from build123d import *

# Parameters (mm, degrees)
F1_DEPTH = 57.15
F2_R     = 10.3251
F3_DEPTH = 7.9375
F4_R     = 9.92251
F5_DEPTH = 88.9


with BuildPart() as f1:
    # F0 (on Right) → F1 (new body)
    with BuildSketch(Plane.YZ):
        with BuildLine():
            Line((-31.75, 0), (0, 0))
            Line((0, 0), (31.75, 0))
            ThreePointArc((31.75, 0), (40.730256, 3.719744), (44.45, 12.7))
            Line((44.45, 12.7), (44.45, 73.025))
            Line((44.45, 73.025), (36.5125, 73.025))
            Line((36.5125, 73.025), (36.5125, 12.7))
            ThreePointArc((36.5125, 12.7), (35.117596, 9.332404), (31.75, 7.9375))
            Line((31.75, 7.9375), (-31.75, 7.9375))
            ThreePointArc((-31.75, 7.9375), (-35.117596, 9.332404), (-36.5125, 12.7))
            Line((-36.5125, 12.7), (-36.5125, 73.025))
            Line((-36.5125, 73.025), (-44.45, 73.025))
            Line((-44.45, 73.025), (-44.45, 12.7))
            ThreePointArc((-44.45, 12.7), (-40.730256, 3.719744), (-31.75, 0))
        make_face()
    extrude(amount=F1_DEPTH)

    # F2 (on face) → F3 (join)
    with BuildSketch(Plane.XY.offset(7.9375)):
        with BuildLine():
            ThreePointArc((63.5, 22.225), (59.009872, 24.084872), (57.15, 28.575))
            Line((57.15, 28.575), (57.15, -28.575))
            ThreePointArc((57.15, -28.575), (59.009872, -24.084872), (63.5, -22.225))
            Line((63.5, -22.225), (111.125, -22.225))
            ThreePointArc((111.125, -22.225), (133.35, 0), (111.125, 22.225))
            Line((111.125, 22.225), (63.5, 22.225))
        make_face()
        with Locations((73.025, 0)):
            Circle(F2_R, mode=Mode.SUBTRACT)
        with Locations((111.125, 0)):
            Circle(F2_R, mode=Mode.SUBTRACT)
    extrude(amount=-F3_DEPTH)

    # F4 (on face) → F5 (cut)
    with BuildSketch(Plane.XZ.offset(44.45)):
        with Locations((28.575, 44.45)):
            Circle(F4_R)
        with BuildLine():
            Line((28.575, 73.025), (0, 73.025))
            Line((0, 73.025), (0, 44.45))
            ThreePointArc((0, 44.45), (8.369424, 64.655576), (28.575, 73.025))
        make_face()
        with BuildLine():
            Line((57.15, 73.025), (28.575, 73.025))
            ThreePointArc((28.575, 73.025), (48.780576, 64.655576), (57.15, 44.45))
            Line((57.15, 44.45), (57.15, 73.025))
        make_face()
    extrude(amount=-F5_DEPTH, mode=Mode.SUBTRACT)


solid = f1.part
Could you check a few things on this model? Use its own coordinates, in mm. A direction names the side the tool comes from. Round coordinates to 2 decimals unless told otherwise and drop trailing zeros. Write each loop counter-clockwise with the first axis right and the second up, starting at its lowest first coordinate (ties: lowest second). Pieces come first, ordered by that corner, then holes. Notation, with made-up numbers: (-26.75, 75.25) -> (32.25, 75.25) arc R13 ccw to (32.25, 82.25) -> close; hole circle Ø7 at (7.25, 61.5). An arc over 180 degrees is marked (long way). Use a Markdown table: item, result.
1. We'd pull the mould along Y, two halves only. Please class faces 4 (the face through (21.8, -44.45, 36.6)), 5 (the face through (22, 44.45, 36)), 6 (the face through (0, -0.6, 7.7)), 7 (the face through (22, -36.512, 36)): +Y half, -Y half, draft (parallel to the pull), parting line (faces both ways), or undercut.
Answer key:
| item | result |
|---|---|
| face 4 | -Y half |
| face 5 | +Y half |
| face 6 | draft |
| face 7 | undercut |
2. If we section it at A-A (z = 22.5): List the corners of the cut face in (x, y) for me, then the cut area to 3 significant figures.
Answer key:
| item | result |
|---|---|
| outline | (0, -44.45) -> (57.15, -44.45) -> (57.15, -36.51) -> (0, -36.51) -> close; (0, 36.51) -> (57.15, 36.51) -> (57.15, 44.45) -> (0, 44.45) -> close |
| area | 907 mm^2 |
3. If we section it at C-C (x = 67.5): List the corners of the cut face in (y, z) for me (1 decimal).
Answer key:
| item | result |
|---|---|
| outline | (-22.2, 0) -> (-8.7, 0) -> (-8.7, 7.9) -> (-22.2, 7.9) -> close; (8.7, 0) -> (22.2, 0) -> (22.2, 7.9) -> (8.7, 7.9) -> close |
4. If we section it at D-D (x = 32): State how many separate pieces and enclosed holes the cut face has, then the cut area to 3 significant figures.
Answer key:
| item | result |
|---|---|
| separate pieces | 3 |
| enclosed holes | 0 |
| area | 1,380 mm^2 |
5. If we section it at B-B (y = 0): List the corners of the cut face in (x, z) for me.
Answer key:
| item | result |
|---|---|
| outline | (0, 0) -> (62.7, 0) -> (62.7, 7.94) -> (0, 7.94) -> close; (83.35, 0) -> (100.8, 0) -> (100.8, 7.94) -> (83.35, 7.94) -> close; (121.45, 0) -> (133.35, 0) -> (133.35, 7.94) -> (121.45, 7.94) -> close |
6. Which directions (+Z, -Z, +X, -X, +Y, -Y) give clear straight access to the entire face, cutting with the end or side of a thin tool? Please do faces 1 (the face through (57.15, 38, 23)), 2 (the face through (57.15, -38, 23)), 3 (the face through (28.175, 35.154, 9.37)).
Answer key:
| item | result |
|---|---|
| face 1 | +Z, -Z, +X, +Y |
| face 2 | +Z, -Z, +X, -Y |
| face 3 | +Z, +X, -X |
7. For pin 1 Ø17.5 at (y, z) = (-36, 12.5) entering from +X; pin 2 Ø4 at (x, z) = (78.5, 4.5) entering from -Y (3 decimals); pin 3 Ø12 at (x, y) = (102, -16) entering from -Z; pin 4 Ø4 at (x, y) = (80.5, 7.5) entering from +Z, each with a flat end and sliding along its axis, tell me the tip position at first contact or that it passes through.
Answer key:
| item | result |
|---|---|
| pin 1 | stops at x = 57.15 |
| pin 2 | stops at y = -22.225 |
| pin 3 | stops at z = 0 |
| pin 4 | stops at z = 7.94 |
8. Please list where these lines run through material, in increasing order: probe 1 along Y at (x, z) = (35, 53.5); probe 2 along Z at (x, y) = (86, 19.5); probe 3 along X at (y, z) = (-37, 38).
Answer key:
| item | result |
|---|---|
| probe 1 | y = -44.45 to -36.51, 36.51 to 44.45 |
| probe 2 | z = 0 to 7.94 |
| probe 3 | x = 0 to 21.03, 36.12 to 57.15 |
